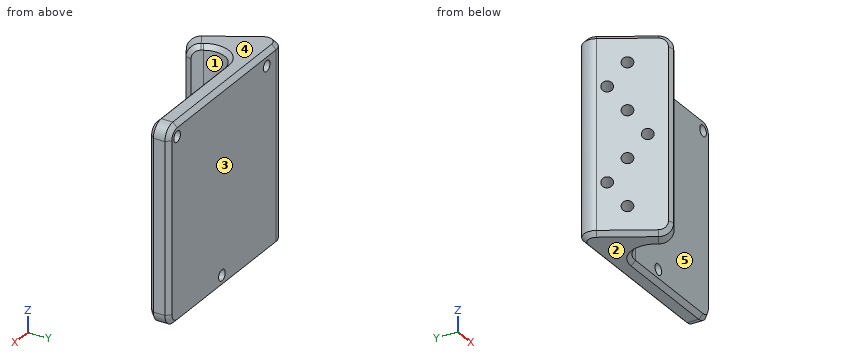
from build123d import *

# Parameters (mm, degrees)
EXTRUDE_1_DEPTH        = 45
FILLET_1_R             = 3
FILLET_2_R             = 5
FILLET_3_R             = 3
FILLET_4_R             = 3
CHAMFER_1_SIZE         = 1
HOLE_WIZARD_M3_1_D     = 2.5
HOLE_WIZARD_M3_1_DEPTH = 7.5
HOLE_WIZARD_M3_1_TIP   = 0.751075774
CHAMFER_2_SIZE         = 1
HOLE_WIZARD_M3_2_D     = 2.5
HOLE_WIZARD_M3_2_DEPTH = 7.5
HOLE_WIZARD_M3_2_TIP   = 0.751075774


with BuildPart() as part:
    # 草图1 → 凸台-拉伸1 (new body)
    with BuildSketch(Plane.XY):
        Polygon((40, 0), (-5.773502692, 0), (4.411675645, -17.641246358), (8.741802661, -15.141246359), (2.685178332, -4.650865298), (40, -4.650865298), align=None)
    extrude(amount=-EXTRUDE_1_DEPTH)

    # 圆角1
    fillet_1_edges = [part.edges().sort_by_distance(p)[0] for p in [
        (40, -2.325432649, -45),
        (40, -2.325432649, 0),
    ]]
    fillet(fillet_1_edges, radius=FILLET_1_R)

    # 圆角2
    fillet_2_edges = [part.edges().sort_by_distance(p)[0] for p in [
        (2.685178332, -4.650865298, -22.5),
    ]]
    fillet(fillet_2_edges, radius=FILLET_2_R)

    # 圆角3
    fillet_3_edges = [part.edges().sort_by_distance(p)[0] for p in [
        (-5.773502692, 0, -22.5),
    ]]
    fillet(fillet_3_edges, radius=FILLET_3_R)

    # 圆角4
    fillet_4_edges = [part.edges().sort_by_distance(p)[0] for p in [
        (6.576739153, -16.391246359, -45),
        (6.576739153, -16.391246359, 0),
    ]]
    fillet(fillet_4_edges, radius=FILLET_4_R)

    # 倒角1
    chamfer_1_edges = [part.edges().sort_by_distance(p)[0] for p in [
        (40, -4.650865298, -22.5),
        (24.172716185, -4.650865298, -45),
        (39.121320344, -4.650865298, -44.121320344),
        (39.121320344, -4.650865298, -0.878679656),
        (7.128554006, -12.347017723, -45),
        (24.172716185, -4.650865298, 0),
        (7.01530535, -7.150865298, 0),
        (7.01530535, -7.150865298, -45),
        (8.741802661, -15.141246359, -22.5),
        (7.128554006, -12.347017723, 0),
        (8.302462833, -14.380287455, -0.878679656),
        (8.302462833, -14.380287455, -44.121320344),
    ]]
    chamfer(chamfer_1_edges, length=CHAMFER_1_SIZE)

    # M3 螺纹孔1
    with Locations(Plane(origin=(0, 0, 0), x_dir=(1, 0, 0), z_dir=(0, 1, 0))):
        with Locations((20, 42), (3, 3), (37, 3)):
            Hole(HOLE_WIZARD_M3_1_D / 2, depth=HOLE_WIZARD_M3_1_DEPTH)
            with Locations((0, 0, -(HOLE_WIZARD_M3_1_DEPTH + HOLE_WIZARD_M3_1_TIP / 2))):  # 118° drill point
                Cone(0, HOLE_WIZARD_M3_1_D / 2, HOLE_WIZARD_M3_1_TIP, mode=Mode.SUBTRACT)

    # 倒角2
    chamfer_2_edges = [part.edges().sort_by_distance(p)[0] for p in [
        (18.211324866, 0, 0),
        (40, 0, -22.5),
        (39.121320344, 0, -44.121320344),
        (39.121320344, 0, -0.878679656),
        (18.211324866, 0, -45),
        (-0.131875417, -9.771585074, 0),
        (-3.17542648, -1.5, 0),
        (-3.17542648, -1.5, -45),
        (-0.131875417, -9.771585074, -45),
        (4.411675645, -17.641246358, -22.5),
        (3.972335817, -16.880287454, -0.878679656),
        (3.972335817, -16.880287454, -44.121320344),
    ]]
    chamfer(chamfer_2_edges, length=CHAMFER_2_SIZE)

    # M3 螺纹孔2
    with Locations(Plane(origin=(-4.330127018, -2.5, 0), x_dir=(0, 0, 1), z_dir=(-0.866025404, -0.5, 0))):
        with Locations((-38.625, -8.3965032), (-33.25, -4.3965032), (-27.875, -8.3965032), (-22.5, -12.3965032), (-17.125, -8.3965032), (-11.75, -4.3965032), (-6.375, -8.3965032)):
            Hole(HOLE_WIZARD_M3_2_D / 2, depth=HOLE_WIZARD_M3_2_DEPTH)
            with Locations((0, 0, -(HOLE_WIZARD_M3_2_DEPTH + HOLE_WIZARD_M3_2_TIP / 2))):  # 118° drill point
                Cone(0, HOLE_WIZARD_M3_2_D / 2, HOLE_WIZARD_M3_2_TIP, mode=Mode.SUBTRACT)


solid = part.part
The listing builds one solid part. Answer for the finished solid, in the listing's coordinates (mm). Face numbers are marked on the shaded views. A direction names the side the tool comes from. Coordinates: 2 decimals unless noted, no trailing zeros. Write each loop counter-clockwise with the first axis right and the second up, starting at its lowest first coordinate (ties: lowest second). Pieces come first, ordered by that corner, then holes. Notation, with made-up numbers: M 33.25,72.5 L 81.25,72.5 A10 cw 81.25,88.5 Z; hole C 55,89 d2. An arc over 180 degrees is marked long. Write each question's results on one line, items separated by ' | '.
Item 1: Which of the six approach directions +Z, -Z, +X, -X, +Y, -Y give full straight-line access (tool end or side, diameter ignored) to the marked faces 4 and 5?
Answer below:
face 4: +Z, +X, -X, +Y, -Y | face 5: +Z, -Z, +X, -Y
Item 2: The part is cut by section A-A on x = 20. Determine the outline of the cut face in (y, z).
Answer below:
outline: M -4.65,-44 L -3.65,-45 L -1,-45 L 0,-44 L 0,-43.25 L -4.65,-43.25 Z; M -4.65,-40.75 L 0,-40.75 L 0,-1 L -1,0 L -3.65,0 L -4.65,-1 Z
Item 3: Given P1, Ø1, axis at x = 7, z = -28.5, coming from the +Y side; P2, Ø3, axis at x = 1.5, z = -7.5, coming from the -Y side; P3, Ø1.5, axis at y = -4.5, z = -21, coming from the -X side; P4, Ø1.5, axis at x = 20, z = -42, coming from the -Y side, each flat-ended and moving along its own axis, determine where each tip first touches the part or whether it passes through.
Answer below:
P1: y = 0 | P2: y = -15.2 | P3: x = -3.48 | P4: through
Item 4: Consider probe 1 along Z at (x, y) = (37, -2.95); probe 2 along Z at (x, y) = (20, -3); probe 3 along Y at (x, z) = (16, -29.5). Determine where each line is inside the solid, lowest interval first. Write a range as [from, to].
Answer below:
probe 1: [-45, -4.25], [-1.75, 0] | probe 2: [-45, -43.25], [-40.75, 0] | probe 3: [-4.65, 0]
Item 5: For a pull along Y with two mould halves and no side action, classify the marked faces 1, 2 and 3 as released by +Y, released by -Y, zero draft, split by the parting line, or undercut.
Answer below:
face 1: undercut | face 2: zero draft | face 3: released by +Y
Item 6: The part is cut by section B-B on z = -36. Determine the outline of the cut face in (x, y).
Answer below:
outline: M -3.18,-4.5 L 3.91,-16.78 L 5.28,-17.14 L 7.88,-15.64 L 8.24,-14.28 L 7.02,-12.15 A5 cw 11.35,-4.65 L 39,-4.65 L 40,-3.65 L 40,-1 L 39,0 L -0.58,0 A3 ccw Z
